Geometry check sheet. Reference: drawing and pictorial views, mm from the part's lowest x, y, z. A direction names the side the tool comes from. Coordinates: 2 decimals unless noted, no trailing zeros. Write each loop counter-clockwise with the first axis right and the second up, starting at its lowest first coordinate (ties: lowest second). Pieces come first, ordered by that corner, then holes. Notation, with made-up numbers: (69.5, 54) -> (121.5, 54) arc R16 cw to (121.5, 74) -> close; hole circle Ø9 at (19, -9.5). An arc over 180 degrees is marked (long way). Use a Markdown table: item, result.
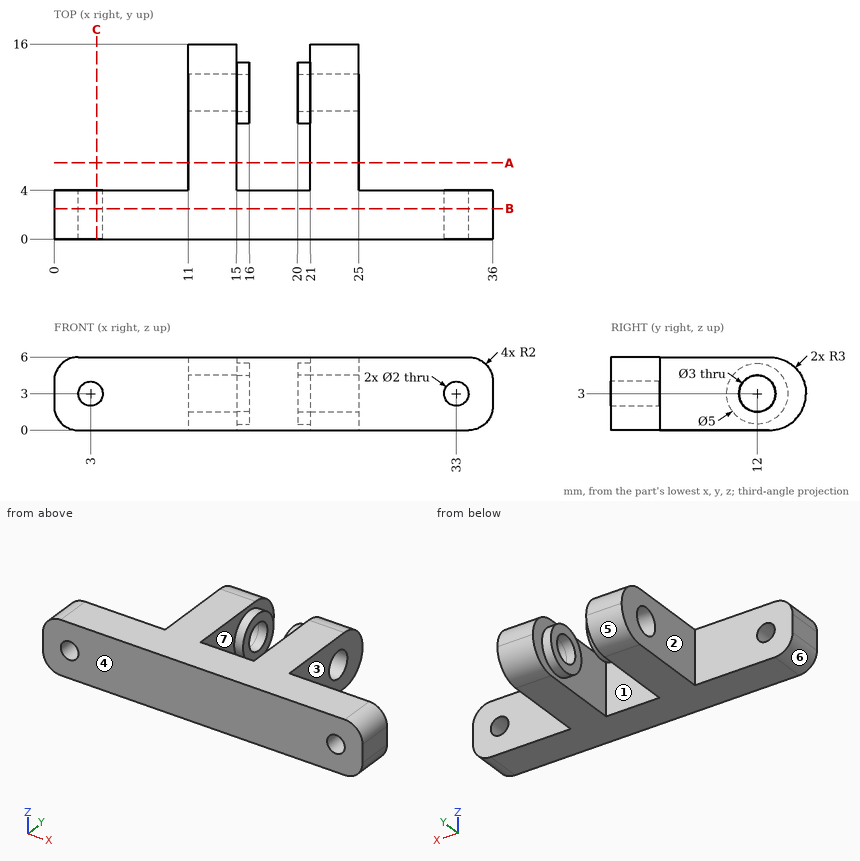
Item 1: Thickness scan on L1, parallel to Y at x = 15.4, z = 3; L2, parallel to Z at x = 12.65, y = 12; L3, parallel to X at y = 5, z = 0.5. Record the ranges inside material, lowest first. Write a range as [from, to].
Answer block:
| item | result |
|---|---|
| L1 | y = [0, 4], [9.5, 10.5], [13.5, 14.5] |
| L2 | z = [0, 1.5], [4.5, 6] |
| L3 | x = [11, 15], [21, 25] |
Item 2: Section check B-B on y = 2.5. Record the boundary of the cut face in (x, z), then the cut area to 3 significant figures.
Answer block:
| item | result |
|---|---|
| outline | (0, 2) arc R2 ccw to (2, 0) -> (34, 0) arc R2 ccw to (36, 2) -> (36, 4) arc R2 ccw to (34, 6) -> (2, 6) arc R2 ccw to (0, 4) -> close; hole circle Ø2 at (3, 3); hole circle Ø2 at (33, 3) |
| area | 206 mm^2 |
Item 3: Section check C-C on x = 3.5. Record the boundary of the cut face in (y, z), then the cut area to 3 significant figures.
Answer block:
| item | result |
|---|---|
| outline | (0, 0) -> (4, 0) -> (4, 2.13) -> (0, 2.13) -> close; (0, 3.87) -> (4, 3.87) -> (4, 6) -> (0, 6) -> close |
| area | 17.1 mm^2 |
Item 4: Mould release check, pull along Y, two halves, no side actions. Record for the marked faces 4, 5, 6 and 7: +Y half, -Y half, draft (parallel to the pull), parting line (faces both ways), or undercut.
Answer block:
| item | result |
|---|---|
| face 4 | -Y half |
| face 5 | +Y half |
| face 6 | draft |
| face 7 | undercut |
Item 5: Section check A-A on y = 6.25. Record the boundary of the cut face in (x, z).
Answer block:
| item | result |
|---|---|
| outline | (11, 0) -> (15, 0) -> (15, 6) -> (11, 6) -> close; (21, 0) -> (25, 0) -> (25, 6) -> (21, 6) -> close |
Item 6: Depth check by flat-ended pin: P1, Ø1.8, axis at x = 7, z = 4, coming from the +Y side; P2, Ø6, axis at x = 28.5, y = 13.5, coming from the -Z side; P3, Ø5, axis at x = 4, y = 4.5, coming from the -Z side; P4, Ø3.5, axis at y = 12, z = 3, coming from the +X side. Enter the tip coordinate at first touch or a pass-through.
Answer block:
| item | result |
|---|---|
| P1 | stops at y = 4 |
| P2 | passes through |
| P3 | stops at z = 0 |
| P4 | stops at x = 25 |
Item 7: Tool access check on the marked faces 1, 2 and 3. Record the directions out of +Z, -Z, +X, -X, +Y, -Y that give a thin tool (end or side, any length) a straight path to the whole face; none if there is none.
Answer block:
| item | result |
|---|---|
| face 1 | +Z, -Z |
| face 2 | +Z, -Z, -X, +Y |
| face 3 | +Z, -Z, +X, +Y |
